Can you work these out from the model? Positions are in its coordinate system, mm. Give positions to 0.01 mm unless a question says otherwise; leave off trailing zeros. Write each loop counter-clockwise with the first axis right and the second up, starting at its lowest first coordinate (ties: lowest second). Pieces come first, ordered by that corner, then holes. Notation, with made-up numbers: M -28.5,28.5 L 7.5,28.5 A35 ccw 7.5,64.5 Z; hole C 20,48.25 d6. An arc over 180 degrees is marked long. Write each question's results on one line, items separated by ' | '.
from build123d import *

# Parameters (mm, degrees)
BOSS_EXTRUDE1_DEPTH     = 304.8
CUT_EXTRUDE1_DEPTH      = 198.18
CUT_EXTRUDE1_DEPTH_BACK = 1
CUT_EXTRUDE4_DEPTH      = 60.305329017


with BuildPart() as part:
    # Sketch1 → Boss-Extrude1 (new body)
    with BuildSketch(Plane(origin=(0, 0, 0), x_dir=(0, 0, -1), z_dir=(1, 0, 0))):
        Polygon((0, 0), (-197.18, 0), (-162.940052328, -59.305329017), align=None)
    extrude(amount=BOSS_EXTRUDE1_DEPTH)

    # Sketch2 → Cut-Extrude1 (cut, two sides)
    with BuildSketch(Plane.XY) as cut_extrude1_sk:
        Polygon((0, 0), (162.940052328, -59.305329017), (0, -59.305329017), align=None)
        Polygon((166.115052328, -59.305329017), (3.175, 0), (304.8, 0), (304.8, -59.305329017), align=None)
    extrude(amount=CUT_EXTRUDE1_DEPTH, mode=Mode.SUBTRACT)
    extrude(cut_extrude1_sk.sketch, amount=-CUT_EXTRUDE1_DEPTH_BACK, mode=Mode.SUBTRACT)

    # Sketch4 → Cut-Extrude4 (cut, through all)
    with BuildSketch(Plane(origin=(0, 0, 0), x_dir=(1, 0, 0), z_dir=(0, 1, 0))):
        Polygon((50.203910812, -187.297424032), (49.714214198, -184.967070242), (0, -195.413931332), (0, -197.18), (3.175, -197.18), align=None)
    extrude(amount=-CUT_EXTRUDE4_DEPTH, mode=Mode.SUBTRACT)


solid = part.part
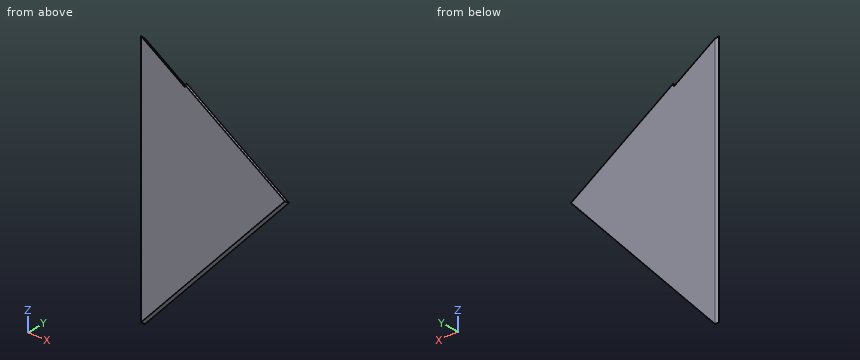
Item 1: If I drill on line 1 (Y direction, x = 37, z = 175.5); line 2 (Y direction, x = 76, z = 141), over which ranges is the centre line in solid material (lowest first)? Write a range as from..to.
Geometry says:
line 1: y = -13.47..-12.31 | line 2: y = -27.66..-26.51
Item 2: I want a section at B-B, the plane z = 178.5. Please give me the cut outline in (x, y) (3 decimals), and give its area (3 significant figures).
Geometry says:
outline: M 0,0 L 88.894,-32.355 L 92.069,-32.355 L 3.175,0 Z | area: 103 mm2
Item 3: I want a section at A-A, the plane y = -14.5. Please give me the cut outline in (x, z).
Geometry says:
outline: M 39.84,39.84 L 43.01,39.84 L 43.01,186.38 L 39.84,187.04 Z
Item 4: I'm going to push flat-ended pins straight in: pin 1 (1 mm diameter, centred on x = 86.5, z = 98, fed in from -Y); pin 2 (5 mm diameter, centred on x = 22.5, y = -7, fed in from +Z); pin 3 (2 mm diameter, centred on x = 108.5, z = 139, fed in from +Y). Where does each tip first touch, or does it pass through?
Geometry says:
pin 1: stops at y = -31.67 | pin 2: stops at z = 191.21 | pin 3: stops at y = -37.97
